Verification items for the finished model (mm, model axes). Face numbers are marked on the shaded views. Give positions to 0.01 mm unless a question says otherwise; leave off trailing zeros. Write each loop counter-clockwise with the first axis right and the second up, starting at its lowest first coordinate (ties: lowest second). Pieces come first, ordered by that corner, then holes. Notation, with made-up numbers: (25, 88) - (60, 88) arc R19 cw to (60, 109) - close; hole circle Ø8 at (15.25, 78). An arc over 180 degrees is marked (long way). Put each result on its own line as item: value.
from build123d import *

# Parameters (mm, degrees)
SKETCH1_R           = 11.5
SKETCH1_R_2         = 2.5
BOSS_EXTRUDE1_DEPTH = 12
CUT_EXTRUDE1_DEPTH  = 12
CIRPATTERN1_COUNT   = 20


with BuildPart() as part:
    # Sketch1 → Boss-Extrude1 (new body)
    with BuildSketch(Plane.XY):
        Circle(SKETCH1_R)
        Circle(SKETCH1_R_2, mode=Mode.SUBTRACT)
    extrude(amount=BOSS_EXTRUDE1_DEPTH)

    # Sketch2 → Cut-Extrude1 (cut)
    with BuildSketch(Plane.XY.offset(12)):
        with BuildLine():
            Line((0, 11.6), (1.5, 11.6))
            Line((1.5, 11.6), (0.8, 10.6))
            Line((0.8, 10.6), (0.559317479, 10))
            ThreePointArc((0.559317479, 10), (0, 9.642447684), (-0.559317479, 10))
            Line((-0.559317479, 10), (-0.8, 10.6))
            Line((-0.8, 10.6), (-1.5, 11.6))
            Line((-1.5, 11.6), (0, 11.6))
        make_face()
    cut_extrude1 = extrude(amount=-CUT_EXTRUDE1_DEPTH, mode=Mode.SUBTRACT)

    # CirPattern1: Cut-Extrude1 ×20 about axis
    cirpattern1_axis = Axis((0, 0, 0), (0, 0, 1))
    for i in range(1, CIRPATTERN1_COUNT):
        add(cut_extrude1.rotate(cirpattern1_axis, i * 360 / CIRPATTERN1_COUNT), mode=Mode.SUBTRACT)


solid = part.part
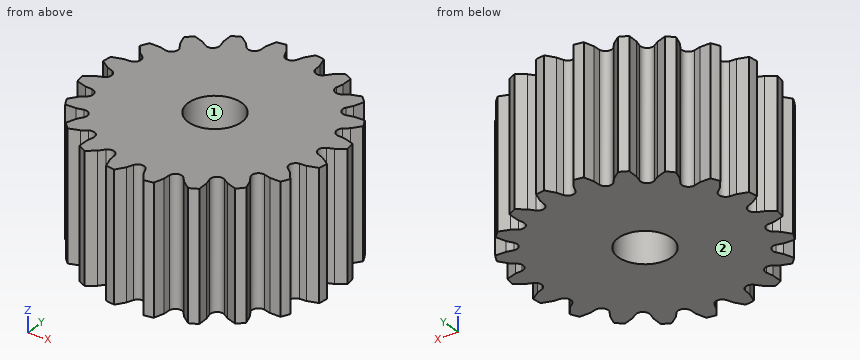
Q1. Go/stop test with flat-tipped pins: pin 1 Ø2 at (x, y) = (-2, -1) entering from +Z; pin 2 Ø6 at (x, z) = (-6.5, 3) entering from +Y; pin 3 Ø3 at (x, y) = (0, 0) entering from +Z; pin 4 Ø1 at (y, z) = (3.5, 10) entering from +X. Record where each tip stops, or that it passes through.
Answers follow:
pin 1: stops at z = 12
pin 2: stops at y = 10.43
pin 3: passes through
pin 4: stops at x = 9.79
Q2. Scan lines: line 1 along X through (y, z) = (10, 1.25); line 2 along X through (y, z) = (-9.25, 1); line 3 along Y through (x, z) = (2, 4.5). Record each from-to range of solid material in increasing order.
Answers follow:
line 1: x = -5.6 to -4.26, -2.54 to -0.56, 0.56 to 2.54, 4.26 to 5.6
line 2: x = -5.59 to -3.52, -2.82 to 2.82, 3.52 to 5.59
line 3: y = -11.32 to -1.5, 1.5 to 11.32
Q3. Section check C-C, the plane x = -3.25. Record the cut outline in (y, z).
Answers follow:
outline: (-9.15, 0) - (9.15, 0) - (9.15, 12) - (-9.15, 12) - close
Q4. Release check for a two-part mould opening along Y. For the marked faces 1 and 2 record: released by +Y, released by -Y, zero draft, split by the parting line, or undercut.
Answers follow:
face 1: undercut
face 2: zero draft
Q5. Section check A-A, the plane y = 0. Record the cut outline in (x, z).
Answers follow:
outline: (-9.64, 0) - (-2.5, 0) - (-2.5, 12) - (-9.64, 12) - close; (2.5, 0) - (9.64, 0) - (9.64, 12) - (2.5, 12) - close
